```python
from build123d import *

# Parameters (mm, degrees)
SKETCH_1_W          = 180
SKETCH_1_H          = 180
SKETCH_1_R          = 1.9
SKETCH_1_R_2        = 75
EXTRUDE_1_DEPTH     = 4
FILLET_1_R          = 10
SKETCH_2_R          = 3
SKETCH_2_R_2        = 2
EXTRUDE_2_DEPTH     = 4
CHAMFER_1_SIZE      = 4
CUT_EXTRUDE_START   = -7
SKETCH_3_R          = 2
CUT_EXTRUDE_1_DEPTH = 7
SKETCH_4_W          = 7
SKETCH_4_H          = 128.601205204
SKETCH_4_W_2        = 130.561529492
SKETCH_4_H_2        = 7
EXTRUDE_3_DEPTH     = 3
FILLET_2_R          = 3


with BuildPart() as part:
    # Эскиз1 → Бобышка-Вытянуть1 (new body)
    with BuildSketch(Plane(origin=(0, 0, 0), x_dir=(1, 0, 0), z_dir=(0, 1, 0))):
        Rectangle(SKETCH_1_W, SKETCH_1_H)
        with Locations(Location((75, 82, 0), (0, 0, 270))):
            Circle(SKETCH_1_R, mode=Mode.SUBTRACT)
        with Locations(Location((82, 75, 0), (0, 0, 270))):
            Circle(SKETCH_1_R, mode=Mode.SUBTRACT)
        with Locations(Location((-82, 75, 0), (0, 0, 90))):
            Circle(SKETCH_1_R, mode=Mode.SUBTRACT)
        with Locations(Location((-75, 82, 0), (0, 0, 90))):
            Circle(SKETCH_1_R, mode=Mode.SUBTRACT)
        with Locations(Location((-82, -75, 0), (0, 0, 270))):
            Circle(SKETCH_1_R, mode=Mode.SUBTRACT)
        with Locations(Location((-75, -82, 0), (0, 0, 270))):
            Circle(SKETCH_1_R, mode=Mode.SUBTRACT)
        with Locations(Location((75, -82, 0), (0, 0, 90))):
            Circle(SKETCH_1_R, mode=Mode.SUBTRACT)
        with Locations(Location((82, -75, 0), (0, 0, 90))):
            Circle(SKETCH_1_R, mode=Mode.SUBTRACT)
        with Locations(Location((0, 0, 0), (0, 0, 270))):
            Circle(SKETCH_1_R_2, mode=Mode.SUBTRACT)
    extrude(amount=EXTRUDE_1_DEPTH)

    # Скругление1
    fillet_1_edges = [part.edges().sort_by_distance(p)[0] for p in [
        (90, 2, 90),
        (-90, 2, 90),
        (-90, 2, -90),
        (90, 2, -90),
    ]]
    fillet(fillet_1_edges, radius=FILLET_1_R)

    # Эскиз2 → Бобышка-Вытянуть2 (add)
    # profile 1 of 4: a face of its own
    with BuildSketch(Plane(origin=(0, 4, 0), x_dir=(1, 0, 0), z_dir=(0, 1, 0))):
        with Locations(Location((-65, 50, 0), (0, 0, 90))):
            Circle(SKETCH_2_R)
        with Locations(Location((-65, 50, 0), (0, 0, 270))):
            Circle(SKETCH_2_R_2, mode=Mode.SUBTRACT)
    # profile 2 of 4: a face of its own
    with BuildSketch(Plane(origin=(0, 4, 0), x_dir=(1, 0, 0), z_dir=(0, 1, 0))):
        with Locations(Location((65, 50, 0), (0, 0, 90))):
            Circle(SKETCH_2_R)
        with Locations(Location((65, 50, 0), (0, 0, 90))):
            Circle(SKETCH_2_R_2, mode=Mode.SUBTRACT)
    # profile 3 of 4: a face of its own
    with BuildSketch(Plane(origin=(0, 4, 0), x_dir=(1, 0, 0), z_dir=(0, 1, 0))):
        with Locations(Location((65, -50, 0), (0, 0, 90))):
            Circle(SKETCH_2_R)
        with Locations(Location((65, -50, 0), (0, 0, 270))):
            Circle(SKETCH_2_R_2, mode=Mode.SUBTRACT)
    # profile 4 of 4: a face of its own
    with BuildSketch(Plane(origin=(0, 4, 0), x_dir=(1, 0, 0), z_dir=(0, 1, 0))):
        with Locations(Location((-65, -50, 0), (0, 0, 90))):
            Circle(SKETCH_2_R)
        with Locations(Location((-65, -50, 0), (0, 0, 90))):
            Circle(SKETCH_2_R_2, mode=Mode.SUBTRACT)
    extrude(amount=EXTRUDE_2_DEPTH)

    # Фаска1
    chamfer_1_edges = [part.edges().sort_by_distance(p)[0] for p in [
        (-65, 4, -47),
        (65, 4, -47),
        (65, 4, 53),
        (-65, 4, 53),
    ]]
    chamfer(chamfer_1_edges, length=CHAMFER_1_SIZE - 0.0001)  # a hair under: the kernel refuses the full size

    # Эскиз3 → Вырез-Вытянуть1 (cut)
    with BuildSketch(Plane(origin=(0, 8, 0), x_dir=(1, 0, 0), z_dir=(0, 1, 0)).offset(CUT_EXTRUDE_START)):
        with Locations(Location((-65, 50, 0), (0, 0, 270))):
            Circle(SKETCH_3_R)
        with Locations(Location((65, 50, 0), (0, 0, 90))):
            Circle(SKETCH_3_R)
        with Locations(Location((65, -50, 0), (0, 0, 270))):
            Circle(SKETCH_3_R)
        with Locations(Location((-65, -50, 0), (0, 0, 90))):
            Circle(SKETCH_3_R)
    extrude(amount=CUT_EXTRUDE_1_DEPTH, mode=Mode.SUBTRACT)

    # Эскиз4 → Бобышка-Вытянуть3 (add)
    with BuildSketch(Plane(origin=(0, 4, 0), x_dir=(1, 0, 0), z_dir=(0, 1, 0))):
        with Locations((-82.5, 0)):
            Rectangle(SKETCH_4_W, SKETCH_4_H)
        with Locations((82.5, 0)):
            Rectangle(SKETCH_4_W, SKETCH_4_H)
        with Locations((0.989102496, -84.539172171)):
            Rectangle(SKETCH_4_W_2, SKETCH_4_H_2)
        with Locations((0.989102496, 82.793697178)):
            Rectangle(SKETCH_4_W_2, SKETCH_4_H_2)
    extrude(amount=EXTRUDE_3_DEPTH)

    # Скругление2
    fillet_2_edges = [part.edges().sort_by_distance(p)[0] for p in [
        (-82.5, 7, 64.300602602),
        (-86, 7, 0),
        (-82.5, 7, -64.300602602),
        (-79, 7, 0),
        (0.989102496, 7, 81.039172171),
        (66.269867242, 7, 84.539172171),
        (0.989102496, 7, 88.039172171),
        (-64.29166225, 7, 84.539172171),
        (82.5, 7, 64.300602602),
        (79, 7, 0),
        (82.5, 7, -64.300602602),
        (86, 7, 0),
        (0.989102496, 7, -79.293697178),
        (-64.29166225, 7, -82.793697178),
        (0.989102496, 7, -86.293697178),
        (66.269867242, 7, -82.793697178),
    ]]
    fillet(fillet_2_edges, radius=FILLET_2_R - 0.0001)  # a hair under: the kernel refuses the full size


solid = part.part
```
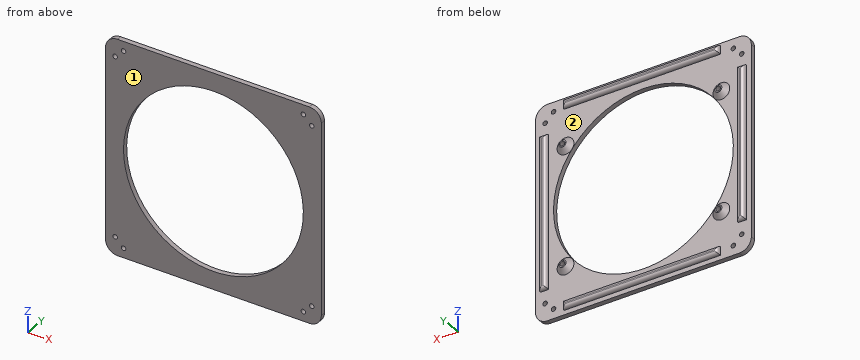
Check sheet for the modelled part. Datum: model origin and axes. Units: mm. Face numbers are marked on the shaded views. A direction names the side the tool comes from. Round coordinates to 2 decimals unless told otherwise and drop trailing zeros. Write item = value, one per line. Start each with the question number.
Q1. Depth check by flat-ended pin: P1, Ø5, axis at x = 65, z = -50, coming from the +Y side; P2, Ø8, axis at x = -52, z = 68, coming from the +Y side; P3, Ø0.8, axis at x = -4.5, z = 84.5, coming from the +Y side; P4, Ø3, axis at y = 7, z = -39, coming from the -X side. Enter the tip coordinate at first touch or a pass-through.
Q2. Access from +Z, -Z, +X, -X, +Y, -Y to the whole of each face (thin tool, end or side, straight path). Record for the marked faces 1 and 2.
Q3. Thickness scan on L1, parallel to X at y = 1.75, z = 76.5; L2, parallel to Y at x = 70, z = -43; L3, parallel to X at y = 2.5, z = -82. Record the ranges inside material, lowest first.
Derived:
q1.P1 = 8
q1.P2 = 4
q1.P3 = 7
q1.P4 = -85.6
q2.face_1 = +Z, -Z, +X, -X, -Y
q2.face_2 = +Y
q3.L1 = -90 to -83.17, -80.83 to 80.83, 83.17 to 90
q3.L2 = 0 to 4
q3.L3 = -89.8 to -76.9, -73.1 to 73.1, 76.9 to 89.8
